Part model, mm, in its own coordinate system. A direction names the side the tool comes from. Round coordinates to 2 decimals unless told otherwise and drop trailing zeros. Order: outer loops, then holes, each group sorted by start corner. A loop starts at its lowest first (then second) coordinate and runs counter-clockwise, first axis right, second up. Notation, with made-up numbers: M 21.25,27 L 59.25,27 A16 cw 59.25,56 Z; hole C 10,33.25 d10. An arc over 180 degrees is marked long. Write each question's results on one line, items separated by ' | '. Start each with the question number.
1. Band-saw the part on A-A, the plane z = 8.5. List the corners of the cut face in (x, y), then the cut area to 3 significant figures.
2. Band-saw the part on C-C, the plane z = 18. List the corners of the cut face in (x, y).
3. Drop a flat-ended pin along its axis: pin 1 Ø1.5 at (y, z) = (1.5, 12) entering from +X. Give the stop position or say it passes through.
4. Two-plate mould, pull along Z, no slides. Class faces 3 (the face through (0, 1, -20)), 4 (the face through (26.99, 1.52, 17.15)), 5 (the face through (-19.152, 2, -11)): +Z half, -Z half, draft (parallel to the pull), parting line (faces both ways), or undercut.
5. Probe L1, parallel to X at y = 1, z = 9.5; L2, parallel to Z at x = 0.5, y = 0.9; L3, parallel to X at y = 1.2, z = -12.5. List the from-to ranges inside material, lowest first. Write a range as [from, to].
6. Band-saw the part on D-D, the plane z = -14. List the corners of the cut face in (x, y).
7. Band-saw the part on B-B, the plane y = 2.45. Give the number of separate pieces and of enclosed holes in the cut face, then the cut area to 3 significant figures.
8. Which spindle directions (+Z, -Z, +X, -X, +Y, -Y) get a long thin tool onto all of the face, cutting with end or side? Do faces 1 (the face through (-10, 2, -16.34)), 2 (the face through (23.591, 2.014, 2.388)). Say none if no direction does.
```python
from build123d import *

# Parameters (mm, degrees)
SKETCH_1_W          = 60
SKETCH_1_H          = 40
EXTRUDE_1_DEPTH     = 3
FILLET_1_R          = 10
SKETCH_2_W          = 1.695959674
SKETCH_2_H          = 10.142260461
CUT_EXTRUDE_1_DEPTH = 4
CUT_EXTRUDE_2_DEPTH = 2
SKETCH_4_R          = 0.5
CUT_EXTRUDE_3_DEPTH = 2


with BuildPart() as part:
    # 草图1 → 凸台-拉伸1 (new body)
    with BuildSketch(Plane(origin=(0, 0, 0), x_dir=(1, 0, 0), z_dir=(0, 1, 0))):
        Rectangle(SKETCH_1_W, SKETCH_1_H)
    extrude(amount=EXTRUDE_1_DEPTH)

    # 圆角1
    fillet_1_edges = [part.edges().sort_by_distance(p)[0] for p in [
        (30, 1.5, 20),
        (-30, 1.5, 20),
        (-30, 1.5, -20),
        (30, 1.5, -20),
    ]]
    fillet(fillet_1_edges, radius=FILLET_1_R)

    # 草图2 → 切除-拉伸1 (cut, through all)
    with BuildSketch(Plane(origin=(0, 3, 0), x_dir=(1, 0, 0), z_dir=(0, 1, 0))):
        with Locations((-20, 11.269178291)):
            Rectangle(SKETCH_2_W, SKETCH_2_H)
        with Locations((-10, 11.269178291)):
            Rectangle(SKETCH_2_W, SKETCH_2_H)
        with Locations((0, 11.269178291)):
            Rectangle(SKETCH_2_W, SKETCH_2_H)
        with Locations((10, 11.269178291)):
            Rectangle(SKETCH_2_W, SKETCH_2_H)
        with Locations((20, 11.269178291)):
            Rectangle(SKETCH_2_W, SKETCH_2_H)
        with Locations((20, -11.269178291)):
            Rectangle(SKETCH_2_W, SKETCH_2_H)
        with Locations((10, -11.269178291)):
            Rectangle(SKETCH_2_W, SKETCH_2_H)
        with Locations((0, -11.269178291)):
            Rectangle(SKETCH_2_W, SKETCH_2_H)
        with Locations((-10, -11.269178291)):
            Rectangle(SKETCH_2_W, SKETCH_2_H)
        with Locations((-20, -11.269178291)):
            Rectangle(SKETCH_2_W, SKETCH_2_H)
    extrude(amount=-CUT_EXTRUDE_1_DEPTH, mode=Mode.SUBTRACT)

    # 草图3 → 切除-拉伸2 (cut)
    with BuildSketch(Plane(origin=(0, 3, 0), x_dir=(1, 0, 0), z_dir=(0, 1, 0))):
        with BuildLine():
            Line((34, 3), (34, -3))
            Line((34, -3), (17, -2))
            ThreePointArc((17, -2), (15, 0), (17, 2))
            Line((17, 2), (34, 3))
        make_face()
    extrude(amount=-CUT_EXTRUDE_2_DEPTH, mode=Mode.SUBTRACT)

    # 草图4 → 切除-拉伸3 (cut, through all)
    with BuildSketch(Plane(origin=(0, 1, 0), x_dir=(1, 0, 0), z_dir=(0, 1, 0))):
        with Locations((16.5, 0)):
            Circle(SKETCH_4_R)
        with Locations((18.5, 0)):
            Circle(SKETCH_4_R)
        with Locations((20.5, 0)):
            Circle(SKETCH_4_R)
        with Locations((22.5, 0)):
            Circle(SKETCH_4_R)
        with Locations((24.5, 0)):
            Circle(SKETCH_4_R)
        with Locations((26.5, 0)):
            Circle(SKETCH_4_R)
        with Locations((28.5, 0)):
            Circle(SKETCH_4_R)
    extrude(amount=-CUT_EXTRUDE_3_DEPTH, mode=Mode.SUBTRACT)


solid = part.part
```
Solution:
1) outline: M -30,0 L -20.85,0 L -20.85,3 L -30,3 Z; M -19.15,0 L -10.85,0 L -10.85,3 L -19.15,3 Z; M -9.15,0 L -0.85,0 L -0.85,3 L -9.15,3 Z; M 0.85,0 L 9.15,0 L 9.15,3 L 0.85,3 Z; M 10.85,0 L 19.15,0 L 19.15,3 L 10.85,3 Z; M 20.85,0 L 30,0 L 30,3 L 20.85,3 Z | area: 155 mm^2
2) outline: M -26,0 L 26,0 L 26,3 L -26,3 Z
3) pin 1: x = 29.92
4) face 3: -Z half | face 4: +Z half | face 5: undercut
5) L1: [-30, -20.85], [-19.15, -10.85], [-9.15, -0.85], [0.85, 9.15], [10.85, 19.15], [20.85, 30] | L2: [-20, -16.34], [-6.2, 6.2], [16.34, 20] | L3: [-29.68, -20.85], [-19.15, -10.85], [-9.15, -0.85], [0.85, 9.15], [10.85, 19.15], [20.85, 29.68]
6) outline: M -29.17,0 L -20.85,0 L -20.85,3 L -29.17,3 Z; M -19.15,0 L -10.85,0 L -10.85,3 L -19.15,3 Z; M -9.15,0 L -0.85,0 L -0.85,3 L -9.15,3 Z; M 0.85,0 L 9.15,0 L 9.15,3 L 0.85,3 Z; M 10.85,0 L 19.15,0 L 19.15,3 L 10.85,3 Z; M 20.85,0 L 29.17,0 L 29.17,3 L 20.85,3 Z
7) separate pieces: 1 | enclosed holes: 10 | area: 2,070 mm^2
8) face 1: +Y, -Y | face 2: +X, +Y
